from build123d import *

# Parameters (mm, degrees)
PAD_DEPTH    = 12
POCKET_DEPTH = 1


with BuildPart() as part:
    # Sketch001 → Pad (new body)
    with BuildSketch(Plane.XZ):
        Polygon((-20, -20), (-20, 110), (136.232082, 151.86226), (292.061476, 580), (480, 511.595971), (480, -20), align=None)
    extrude(amount=-PAD_DEPTH)

    # Sketch002 (on Face7 of Pad) → Pocket (cut)
    with BuildSketch(Plane.XZ):
        Polygon((465, -5), (465, 501.092858), (301.026563, 560.774309), (147.656805, 139.394363), (-5, 98.490095), (-5, -5), align=None)
    extrude(amount=POCKET_DEPTH, mode=Mode.SUBTRACT)


solid = part.part
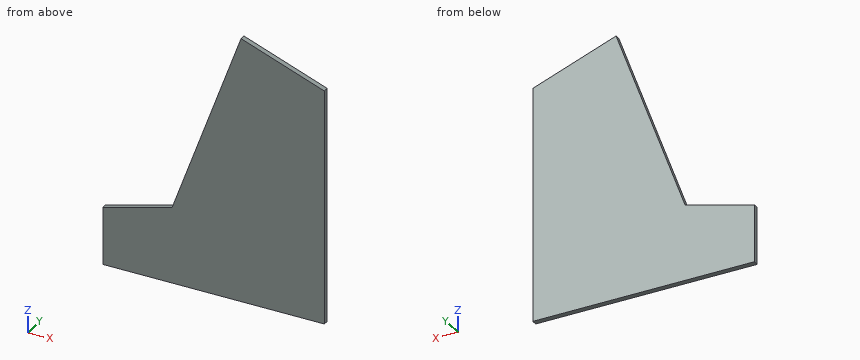
Geometry: final body of the model. Coordinates: model frame, mm. Round coordinates to 2 decimals unless told otherwise and drop trailing zeros. Loops run counter-clockwise (first coordinate to the right, second up) from the corner with the lowest first, then second, coordinate; pieces in that order, holes last. Notation, with made-up numbers: M -1,38 L 36,38 A22 ccw 36,64 Z; hole C 46,42 d7. An arc over 180 degrees is marked long. One line per question, with ' | ' between items.
(1) Cut plane B-B on x = 323.5. Return the cut outline in (y, z), plus the area to 3 significant figures.
Check result:
outline: M 0,-20 L 12,-20 L 12,568.56 L 0,568.56 Z | area: 7,060 mm2
(2) Cut plane A-A on y = 8.5. Return the cut outline in (x, z).
Check result:
outline: M -20,-20 L 480,-20 L 480,511.6 L 292.06,580 L 136.23,151.86 L -20,110 Z
(3) Cut plane C-C on z = 365. Return the cut outline in (x, y).
Check result:
outline: M 213.81,0 L 480,0 L 480,12 L 213.81,12 Z
(4) Material intervals for line 1 along X through (y, z) = (3, 195); line 2 along Z through (x, y) = (111, 2.25); line 3 along Z through (x, y) = (300, 2.25), sorted ascending. Write a range as from..to.
Check result:
line 1: x = 151.93..480 | line 2: z = -20..145.1 | line 3: z = -20..577.11
(5) Contact query for a flat-ended pin moving along its axis: P1, Ø3, axis at y = 5.5, z = 233.5, coming from the -X side. Output: stop coordinate, or through.
Check result:
P1: stops at x = 165.4
